Autodesk Fusion 360 part; units mm, degrees
sketch "Sketch1" plane through (0, 0, 0) normal (0, 1, 0) x (1, 0, 0)
  circle A0 centre (0, 0) radius 7.5
  line L0 (6.4897, 0.2677) -> (3.013, 5.7541)
  line L1 (3.013, 5.7541) -> (-3.4767, 5.4864)
  line L2 (-3.4767, 5.4864) -> (-6.4897, -0.2677)
  line L3 (-6.4897, -0.2677) -> (-3.013, -5.7541)
  line L4 (-3.013, -5.7541) -> (3.4767, -5.4864)
  line L5 (3.4767, -5.4864) -> (6.4897, 0.2677)
  circle A1 centre (0, 0) radius 3.55
  dimension "d1" = 15
  dimension "d2" = 5.625
  dimension "d7" = 7.1
extrude "Extrude1" add sketch "Sketch1" along normal blind 42.88 contours A0 | L0 L1 L2 L3 L4 L5 | A1
extrude "Extrude2" cut sketch "Sketch1" along normal blind 5.9 contours L0 L1 L2 L3 L4 L5 | A1
extrude "Extrude3" cut sketch "Sketch1" along normal blind 39 contours A1
sketch "Sketch2" plane through (0, 42.88, 0) normal (0, 1, 0) x (-1, 0, 0)
  circle A0 centre (0, 0) radius 7.5
  circle A1 centre (0, 0) radius 3.98
  dimension "d10" = 7.96
extrude "Extrude4" add sketch "Sketch2" along normal blind 5.8 contours A1
fillet "Fillet1" radius 0.4 1 edges at (3.7107, 48.68, -1.4392)
The model under review builds one solid part; all positions refer to its coordinate system, in mm. A direction names the side the tool comes from. Round coordinates to 2 decimals unless told otherwise and drop trailing zeros. Loops run counter-clockwise (first coordinate to the right, second up) from the corner with the lowest first, then second, coordinate; pieces in that order, holes last. Notation, with made-up numbers: (-37, 28.5) - (-23, 28.5) arc R7 ccw to (-23, 34.5) - close; hole circle Ø9 at (69.25, 87.25). An arc over 180 degrees is marked (long way). Use CSV: the item, a comma, the result in double quotes.
(1) Machinability: for faces 5 (the flat face through (3, 42.88, 3)), 6 (the flat face through (-4.96, 2.91, -2.65)), 7 (the cylindrical face through (-7.493, 21.14, 0.33)), which of the approach directions +Z, -Z, +X, -X, +Y, -Y give a long, thin tool a straight path to every point of the face, cutting with its end or side? Answer none if there is none.
Working result:
face 5,"+Y"
face 6,"-Y"
face 7,"+Y, -Y"
(2) For line 1 (X direction, y = 19.5, z = 0); line 2 (Y direction, x = 3.25, z = -4.5), list the stretches that pass through material, from the lowest coordinate up.
Working result:
line 1,"x = -7.5 to -3.55, 3.55 to 7.5"
line 2,"y = 5.9 to 42.88"
(3) Take a section at B-B, the plane z = 5. Give the boundary of the cut face in (x, y).
Working result:
outline,"(-5.59, 0) - (-3.49, 0) - (-3.49, 5.9) - (3.73, 5.9) - (3.73, 0) - (5.59, 0) - (5.59, 42.88) - (-5.59, 42.88) - close"
(4) The part is to be moulded in two halves that separate along X. For faces 1 (the flat face through (2.8, 5.9, 2.5)), 2 (the flat face through (-5, 0, -3)), 3 (the cylindrical face through (0.518, 45.542, -3.946)), 4 (the flat face through (-4.776, 2.909, 2.972)), say which applies: pulls with the +X half, pulls with the -X half, needs draft (parallel to the pull), parting line crosses it, or undercut.
Working result:
face 1,"undercut"
face 2,"needs draft"
face 3,"parting line crosses it"
face 4,"undercut"
(5) Clearance check with flat-ended pins moving along their axes: P1, Ø4, axis at x = -2.5, y = 13.5, coming from the -Z side; P2, Ø1.5, axis at x = -4.5, y = 14, coming from the -Z side; P3, Ø8, axis at x = -1.5, z = -5, coming from the +Y side; P4, Ø2, axis at x = -4, y = 34, coming from the +Z side. State where each tip first meets the part, or that it passes through.
Working result:
P1,"stops at z = -7.48"
P2,"stops at z = -6.5"
P3,"stops at y = 48.68"
P4,"stops at z = 6.87"
(6) Take a section at D-D, the plane y = 40. Give the boundary of the cut face in (x, z), plus the area to 3 significant figures.
Working result:
outline,"circle Ø15 at (0, 0)"
area,"177 mm^2"
(7) Take a section at C-C, the plane y = 27. Give the boundary of the cut face in (x, z).
Working result:
outline,"circle Ø15 at (0, 0); hole circle Ø7.1 at (0, 0)"
(8) Take a section at A-A, the plane x = -5. Give the boundary of the cut face in (y, z).
Working result:
outline,"(0, -5.59) - (42.88, -5.59) - (42.88, 5.59) - (0, 5.59) - (0, 2.62) - (5.9, 2.62) - (5.9, -2.58) - (0, -2.58) - close"
